Geometry check sheet. Reference: the model listing, model coordinates, mm. A direction names the side the tool comes from. Round coordinates to 2 decimals unless told otherwise and drop trailing zeros. Order: outer loops, then holes, each group sorted by start corner. A loop starts at its lowest first (then second) coordinate and runs counter-clockwise, first axis right, second up.
```python
from build123d import *

# Parameters (mm, degrees)
SKETCH1_R                      = 12.7
BOSS_EXTRUDE1_DEPTH            = 5.08
SKETCH2_R                      = 6.096
BOSS_EXTRUDE2_DEPTH            = 4.064
SKETCH3_R                      = 3
CUT_EXTRUDE1_DEPTH             = 21.154223776
SKETCH7_W                      = 1.1303
SKETCH7_H                      = 12.7
F_4_40_TAPPED_HOLE1_AT_2_COUNT = 2
F_4_40_TAPPED_HOLE1_AT_2_PITCH = 4.572
F_4_40_TAPPED_HOLE2_D          = 2.2606


with BuildPart() as part:
    # Sketch1 → Boss-Extrude1 (new body)
    with BuildSketch(Plane(origin=(0, 0, 0), x_dir=(1, 0, 0), z_dir=(0, 1, 0))):
        with Locations(Location((0, 0, 0), (0, 0, 270))):
            Circle(SKETCH1_R)
    extrude(amount=BOSS_EXTRUDE1_DEPTH)

    # Sketch2 → Boss-Extrude2 (add)
    with BuildSketch(Plane(origin=(0, 5.08, 0), x_dir=(1, 0, 0), z_dir=(0, 1, 0))):
        with Locations(Location((0, 0, 0), (0, 0, 270))):
            Circle(SKETCH2_R)
    extrude(amount=BOSS_EXTRUDE2_DEPTH)

    # Sketch3 → Cut-Extrude1 (cut, through all)
    with BuildSketch(Plane(origin=(0, 9.144, 0), x_dir=(1, 0, 0), z_dir=(0, 1, 0))):
        with Locations(Location((0, 0, 0), (0, 0, 270))):
            Circle(SKETCH3_R)
    extrude(amount=-CUT_EXTRUDE1_DEPTH, mode=Mode.SUBTRACT)

    # Sketch7 → #4-40 Tapped Hole1 (revolve, cut)
    with BuildSketch(Plane(origin=(0, 7.112, 0), x_dir=(0, 1, 0), z_dir=(1, 0, 0))):
        with Locations((0.56515, 6.35)):
            Rectangle(SKETCH7_W, SKETCH7_H)
    f_4_40_tapped_hole1 = revolve(axis=Axis((0, 7.112, -6.35), (0, 0, 1)), mode=Mode.SUBTRACT)

    # #4-40 Tapped Hole1 at 2: #4-40 Tapped Hole1 ×2
    with Locations(*[(0, -i * F_4_40_TAPPED_HOLE1_AT_2_PITCH, 0) for i in range(1, F_4_40_TAPPED_HOLE1_AT_2_COUNT)]):
        add(f_4_40_tapped_hole1, mode=Mode.SUBTRACT)

    # #4-40 Tapped Hole2 (through all)
    with Locations(Plane(origin=(0, 0, 0), x_dir=(-1, 0, 0), z_dir=(0, -1, 0))):
        with Locations((9.525, 0), (4.7625, -8.248891971), (-4.7625, -8.248891971), (-9.525, 0), (-4.7625, 8.248891971), (4.7625, 8.248891971)):
            Hole(F_4_40_TAPPED_HOLE2_D / 2)


solid = part.part
```
(1) Draft check along Y on faces 1 (the flat face through (-3, 0, 3)), 2 (the cylindrical face through (5.84, 2.58, -8.59)), 3 (the cylindrical face through (0.433, 8.156, 4.461)). Enter one of: released by +Y, released by -Y, zero draft, split by the parting line, or undercut.
Returned:
face 1: released by -Y
face 2: zero draft
face 3: undercut
(2) Material ranges on line 1 (Y direction, x = 0, z = 9); line 2 (X direction, y = 3, z = 0.25); line 3 (Z direction, x = 5.25, y = 1), recorded low to high.
Returned:
line 1: y = 0 to 1.41, 3.67 to 5.08
line 2: x = -12.7 to -10.63, -8.42 to -2.99, 2.99 to 8.42, 10.63 to 12.7
line 3: z = -11.56 to -9.27, -7.23 to 7.23, 9.27 to 11.56
(3) Sectioned sample at D-D, the plane x = 5.5. Record the cut outline in (y, z).
Returned:
outline: (0, -11.45) - (5.08, -11.45) - (5.08, -9.11) - (0, -9.11) - close; (0, -7.39) - (5.08, -7.39) - (5.08, -2.63) - (9.14, -2.63) - (9.14, 2.63) - (5.08, 2.63) - (5.08, 7.39) - (0, 7.39) - close; (0, 9.11) - (5.08, 9.11) - (5.08, 11.45) - (0, 11.45) - close
(4) Sectioned sample at C-C, the plane y = 2.54. Record the cut outline in (x, z) (1 decimal).
Returned:
outline: (-1.1, 2.8) - (-1.1, 12.6) arc R12.7 ccw (long way) to (1.1, 12.6) - (1.1, 2.8) arc R3 cw (long way) to start; hole circle Ø2.3 at (-9.5, 0); hole circle Ø2.3 at (-4.8, -8.2); hole circle Ø2.3 at (-4.8, 8.2); hole circle Ø2.3 at (4.8, -8.2); hole circle Ø2.3 at (4.8, 8.2); hole circle Ø2.3 at (9.5, 0)
(5) Set-up check for faces 4 (the cylindrical face through (-10.654, 2.576, -0.05)), 5 (the cylindrical face through (0.433, 3.584, 7.809)), 6 (the flat face through (-5.5, 5.08, -3)): record each of +Z, -Z, +X, -X, +Y, -Y from which the full face is reachable in a straight line by a thin tool's end or side.
Returned:
face 4: +Y, -Y
face 5: +Z
face 6: +Y
(6) Sectioned sample at A-A, the plane x = 0. Record the cut outline in (y, z).
Returned:
outline: (0, -12.7) - (5.08, -12.7) - (5.08, -6.1) - (9.14, -6.1) - (9.14, -3) - (0, -3) - close; (0, 3) - (1.41, 3) - (1.41, 12.7) - (0, 12.7) - close; (3.67, 3) - (5.98, 3) - (5.98, 6.1) - (5.08, 6.1) - (5.08, 12.7) - (3.67, 12.7) - close; (8.24, 3) - (9.14, 3) - (9.14, 6.1) - (8.24, 6.1) - close
(7) Depth check by flat-ended pin: P1, Ø3, axis at x = -4.76, z = -8.25, coming from the +Y side; P2, Ø3.5, axis at x = 0, y = 2.54, coming from the +Z side; P3, Ø3, axis at x = 0, y = 7.112, coming from the -Z side; P4, Ø1, axis at x = -8, y = 4.5, coming from the -Z side. Enter the tip coordinate at first touch or a pass-through.
Returned:
P1: stops at y = 5.08
P2: stops at z = 12.7
P3: stops at z = -6.1
P4: stops at z = -10.25
(8) Sectioned sample at B-B, the plane z = 0. Record the cut outline in (x, y).
Returned:
outline: (-12.7, 0) - (-10.66, 0) - (-10.66, 5.08) - (-12.7, 5.08) - close; (-8.39, 0) - (-3, 0) - (-3, 9.14) - (-6.1, 9.14) - (-6.1, 5.08) - (-8.39, 5.08) - close; (3, 0) - (8.39, 0) - (8.39, 5.08) - (6.1, 5.08) - (6.1, 9.14) - (3, 9.14) - close; (10.66, 0) - (12.7, 0) - (12.7, 5.08) - (10.66, 5.08) - close
